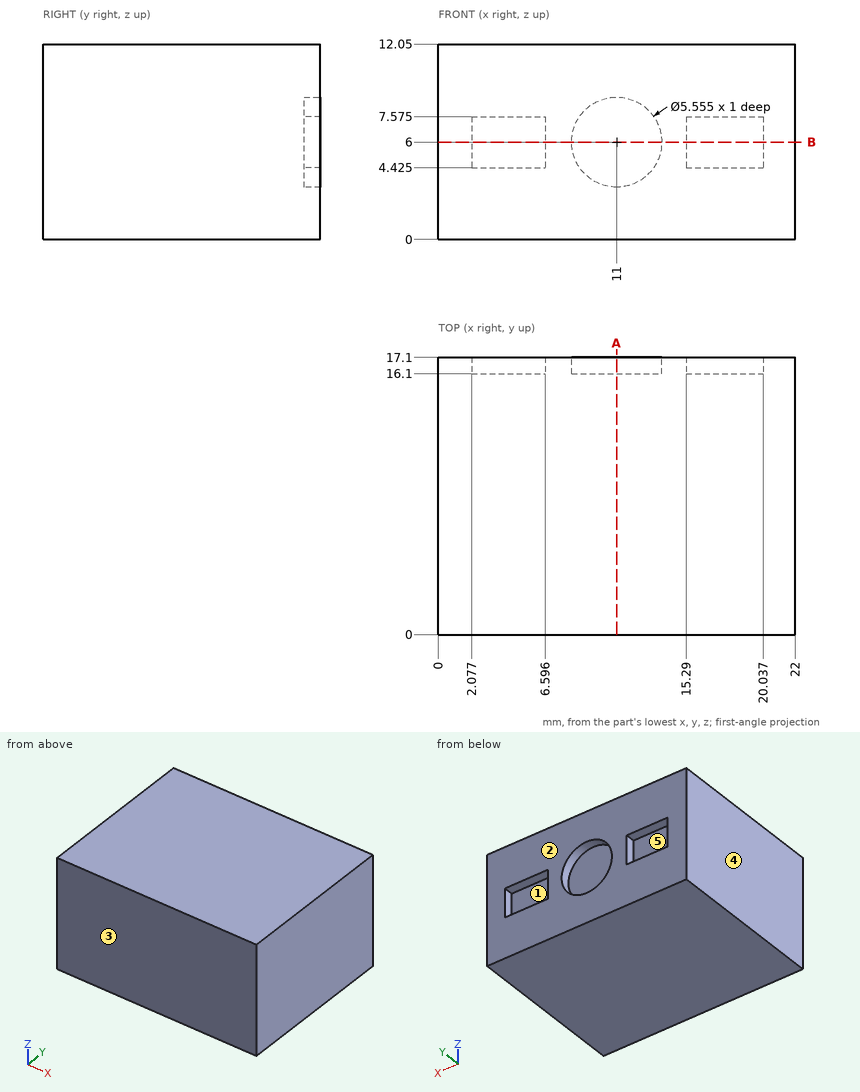
Job drawing, mm, ordinate dimensions from the low corner. One solid piece. A direction names the side the tool comes from. Coordinates: 2 decimals unless noted, no trailing zeros. Write each loop counter-clockwise with the first axis right and the second up, starting at its lowest first coordinate (ties: lowest second). Pieces come first, ordered by that corner, then holes.
Item 1: Pin check, flat tip, straight feed: pin 1 (0.9 mm diameter, centred on x = 16.5, z = 6.5, fed in from +Y). Stop position of the tip, or through.
Item 2: Mould opens along X. For the marked faces 3, 4 and 5 say: released by +X, released by -X, zero draft, split by the parting line, or undercut.
Item 3: Slice it at A-A (x = 11). Write the cut outline in (y, z).
Item 4: Slice it at B-B (z = 6). Write the cut outline in (x, y) (1 decimal), and give its area (3 significant figures).
Item 5: Probe line 1 (X direction, y = 16.45, z = 6) (1 decimal); line 2 (Z direction, x = 11, y = 16.7); line 3 (Y direction, x = 5, z = 5). List the from-to ranges inside material, lowest first.
Item 6: Which spindle directions (+Z, -Z, +X, -X, +Y, -Y) get a long thin tool onto all of the face, cutting with end or side? Do the marked faces 1 and 2. Say none if no direction does.
Results found:
1. pin 1: stops at y = 16.1
2. face 3: zero draft
2. face 4: released by -X
2. face 5: undercut
3. outline: (0, 0) - (17.1, 0) - (17.1, 3.22) - (16.1, 3.22) - (16.1, 8.78) - (17.1, 8.78) - (17.1, 12.05) - (0, 12.05) - close
4. outline: (0, 0) - (22, 0) - (22, 17.1) - (20, 17.1) - (20, 16.1) - (15.3, 16.1) - (15.3, 17.1) - (13.8, 17.1) - (13.8, 16.1) - (8.2, 16.1) - (8.2, 17.1) - (6.6, 17.1) - (6.6, 16.1) - (2.1, 16.1) - (2.1, 17.1) - (0, 17.1) - close
4. area: 361 mm2
5. line 1: x = 0 to 2.1, 6.6 to 8.2, 13.8 to 15.3, 20 to 22
5. line 2: z = 0 to 3.22, 8.78 to 12.05
5. line 3: y = 0 to 16.1
6. face 1: +Y
6. face 2: +Z, -Z, +X, -X, +Y
